```python
from build123d import *

# Parameters (mm, degrees)
PAD_DEPTH       = 90
SKETCH_R        = 5
SKETCH_R_2      = 1.5
SKETCH_R_3      = 10.4
POCKET_DEPTH    = 95
POCKET001_DEPTH = 32
SKETCH005_W     = 23
SKETCH005_H     = 23
POCKET002_DEPTH = 20
SKETCH006_W     = 23
SKETCH006_H     = 23
POCKET003_DEPTH = 20


with BuildPart() as part:
    # Sketch003 → Pad (new body)
    with BuildSketch(Plane.XY.offset(100)):
        Polygon((7.5, 0), (0, 0), (0, -30), (95, -30), (95, -0.086413), (87.5, -0.086413), (87.5, 2), (90.2, 2), (87, 5.2), (83, 5.2), (79.8, 2), (82.5, 2), (82.5, -0.086413), (12.5, -0.086413), (12.5, 2), (15.2, 2), (12, 5.2), (8, 5.2), (4.8, 2), (7.5, 2), align=None)
    extrude(amount=PAD_DEPTH)

    # Sketch (on Face4 of Pad) → Pocket (cut)
    with BuildSketch(Plane(origin=(95, 0, 100), x_dir=(0, 1, 0), z_dir=(1, 0, 0))):
        with Locations((-15, 45)):
            Circle(SKETCH_R)
        with Locations((-15, 52.5)):
            Circle(SKETCH_R_2)
        with Locations((-22.5, 45)):
            Circle(SKETCH_R_2)
        with Locations((-15, 37.5)):
            Circle(SKETCH_R_2)
        with Locations((-7.5, 45)):
            Circle(SKETCH_R_2)
        with Locations((-15, 20.5)):
            Circle(SKETCH_R_3)
        with Locations((-15, 69.5)):
            Circle(SKETCH_R_3)
    extrude(amount=-POCKET_DEPTH, mode=Mode.SUBTRACT)

    # Sketch004 (on Face7 of Pocket) → Pocket001 (cut)
    with BuildSketch(Plane(origin=(0, -30, 100), x_dir=(1, 0, 0), z_dir=(0, -1, 0))):
        with BuildLine():
            Line((30, 80.681485), (30, 64.654132))
            ThreePointArc((30, 64.654132), (31.683486, 60.589837), (35.747781, 58.906351))
            Line((35.747781, 58.906351), (58.899356, 58.906351))
            ThreePointArc((58.899356, 58.906351), (63.213163, 60.693188), (65, 65.006995))
            Line((65, 80.523747), (65, 65.006995))
            ThreePointArc((65, 80.523747), (63.688936, 83.688936), (60.523747, 85))
            Line((34.318515, 85), (60.523747, 85))
            ThreePointArc((34.318515, 85), (31.264864, 83.735136), (30, 80.681485))
        make_face()
        with BuildLine():
            Line((34.00557, 30.656874), (60.341932, 30.656874))
            ThreePointArc((64.957016, 26.04179), (63.605289, 29.305147), (60.341932, 30.656874))
            Line((64.957016, 8.697674), (64.957016, 26.04179))
            ThreePointArc((61.259342, 5), (63.873992, 6.083024), (64.957016, 8.697674))
            Line((33.329898, 5), (61.259342, 5))
            ThreePointArc((29.898488, 8.43141), (30.903525, 6.005037), (33.329898, 5))
            Line((29.898488, 8.43141), (29.898488, 26.549793))
            ThreePointArc((34.00557, 30.656874), (31.101424, 29.453938), (29.898488, 26.549793))
        make_face()
    extrude(amount=-POCKET001_DEPTH, mode=Mode.SUBTRACT)

    # Sketch005 (on Face3 of Pocket001) → Pocket002 (cut)
    with BuildSketch(Plane(origin=(0, 0, 100), x_dir=(0, -1, 0), z_dir=(-1, 0, 0))):
        with Locations((15, 45)):
            Rectangle(SKETCH005_W, SKETCH005_H)
    extrude(amount=-POCKET002_DEPTH, mode=Mode.SUBTRACT)

    # Sketch006 (on Face14 of Pocket002) → Pocket003 (cut)
    with BuildSketch(Plane(origin=(95, 0, 100), x_dir=(0, 1, 0), z_dir=(1, 0, 0))):
        with Locations((-15, 45)):
            Rectangle(SKETCH006_W, SKETCH006_H)
    extrude(amount=-POCKET003_DEPTH, mode=Mode.SUBTRACT)


solid = part.part
```
Input: part model. Units: mm. Frame: model coordinates. A direction names the side the tool comes from. Coordinates: 2 decimals unless noted, no trailing zeros. Order: outer loops, then holes, each group sorted by start corner. A loop starts at its lowest first (then second) coordinate and runs counter-clockwise, first axis right, second up. Notation, with made-up numbers: (5.5, 20.5) - (29.5, 20.5) arc R13 cw to (29.5, 39.5) - close; hole circle Ø7 at (71, 52.25). An arc over 180 degrees is marked (long way). Return JSON: item names as keys, results as strings.
Q1. Cut plane C-C (z = 169.5). State how many separate pieces and enclosed holes the cut face has, then the cut area to 3 significant figures.
The answers:
{"separate pieces": "4", "enclosed holes": "0", "area": "614 mm2"}
Q2. Draft query along X for faces 1 (the cylindrical face through (48, -15, 154)), 2 (the flat face through (48, -0.086, 144)), 3 (the flat face through (88.6, 3.6, 144.4)). Return one class per face: +X half, -X half, draft (parallel to the pull), parting line (faces both ways), or undercut.
The answers:
{"face 1": "draft", "face 2": "undercut", "face 3": "+X half"}
Q3. Ray query, probe 1 along Z at (x, y) = (88, -15); probe 2 along X at (y, z) = (-1.5, 110); probe 3 along Z at (x, y) = (36.5, -4). Return the intervals inside material, ascending.
The answers:
{"probe 1": "z = 100 to 110.1, 130.9 to 133.5, 156.5 to 159.1, 179.9 to 190", "probe 2": "x = 0 to 29.9, 64.96 to 95", "probe 3": "z = 100 to 105, 130.66 to 158.91, 185 to 190"}
Q4. Cut plane B-B (x = 47.5). Return loops of the section in (y, z), then the cut area to 3 significant figures.
The answers:
{"outline": "(-30, 100) - (-0.09, 100) - (-0.09, 105) - (-30, 105) - close; (-30, 130.66) - (-17.24, 130.66) arc R10.4 cw to (-12.76, 130.66) - (-0.09, 130.66) - (-0.09, 158.91) - (-30, 158.91) - close; (-30, 185) - (-0.09, 185) - (-0.09, 190) - (-30, 190) - close; hole circle Ø3 at (-22.5, 145); hole circle Ø10 at (-15, 145); hole circle Ø3 at (-15, 137.5); hole circle Ø3 at (-15, 152.5); hole circle Ø3 at (-7.5, 145)", "area": "1,040 mm2"}
Q5. First-contact query: pin 1 (0.6 mm diameter, centred on y = 0.5, z = 132.5, fed in from -X); pin 2 (8 mm diameter, centred on x = 2.5, z = 128.5, fed in from +Y); pin 3 (12 mm diameter, centred on y = -12.5, z = 144, fed in from -X); pin 4 (12.5 mm diameter, centred on y = -15, z = 120.5, fed in from +X). Flat tips, straight axial feed; report the tip coordinate or a pass-through.
The answers:
{"pin 1": "stops at x = 7.5", "pin 2": "stops at y = 3.7", "pin 3": "stops at x = 20", "pin 4": "passes through"}
Q6. Access query for faces 4 (the flat face through (6, 2, 144)), 5 (the flat face through (85, -15, 156.5)), 6 (the flat face through (29.898, -15, 109)), 7 (the flat face through (81, 2, 144)). Directions: +Z, -Z, +X, -X, +Y, -Y. A direction counts if a zero-diameter tool reaches every point of the face in a straight line with its end or side. Return the directions, or none.
The answers:
{"face 4": "+Z, -Z, -X", "face 5": "+X", "face 6": "+Y, -Y", "face 7": "+Z, -Z"}
